Model file for the job. Use its own axes, mm. A direction names the side the tool comes from. Coordinates: 2 decimals unless noted, no trailing zeros. Write each loop counter-clockwise with the first axis right and the second up, starting at its lowest first coordinate (ties: lowest second). Pieces come first, ordered by that corner, then holes. Notation, with made-up numbers: (19.25, 77) - (78.25, 77) arc R27 ccw to (78.25, 109) - close; hole circle Ø7 at (-31.5, 2). An arc over 180 degrees is marked (long way). Put each result on its own line as item: value. Start each with the question number.
1. Saw through at B-B, the plane x = -24. Write the cut outline in (y, z).
2. Which spindle directions (+Z, -Z, +X, -X, +Y, -Y) get a long thin tool onto all of the face, cutting with end or side? Do faces 1 (the face through (2, -7, -5.2)), 2 (the face through (0, 124.252, 0)). Say none if no direction does.
3. Saw through at A-A, the plane z = -3. Write the cut outline in (x, y), plus the area to 3 significant figures.
4. Drill centre lines: L1, parallel to Z at x = 49, y = -55; L2, parallel to X at y = -49, z = -1.75; L3, parallel to X at y = 69.5, z = -2.25. Where is each one in solid material? Low to high. Write a range as from..to.
5. Saw through at C-C, the plane y = 107.5. Write the cut outline in (x, z).
6. Pull direction Z, two halves, no side cores. Call faces 3 (the face through (-79.427, 62.996, 0.08)), 4 (the face through (0, 123.744, 0)), 5 (the face through (-2, -7, 5.708)): released by +Z, released by -Z, zero draft, split by the parting line, or undercut.
7. Drop flat-ended pins along their axis: P1, Ø1, axis at x = -26, z = 3.5, coming from the +Y side; P2, Ø5, axis at x = -104.5, z = -3, coming from the -Y side; P3, Ø0.6, axis at y = 124, z = 4.5, coming from the -X side. Give the stop position or say it passes through.
Autodesk Inventor part; units mm, degrees
ref_plane "YZ Plane" through (0, 0, 0) normal (1, 0, 0) x (0, 1, 0)
ref_plane "XZ Plane" through (0, 0, 0) normal (0, 1, 0) x (-1, 0, 0)
ref_plane "XY Plane" through (0, 0, 0) normal (0, 0, 1) x (1, 0, 0)
sketch "Sketch1" plane through (0, 0, 0) normal (0, 0, 1) x (1, 0, 0)
  line L0 (-141.7042, 0) -> (-17.9605, 123.7437)
  line L1 (17.9605, 123.7437) -> (141.7042, 0)
  line L2 (141.7042, 0) -> (0, -141.7042)
  line L3 (0, -141.7042) -> (-141.7042, 0)
  line L4 (-141.7042, 0) -> (141.7042, 0) construction
  line L5 (0, 141.7042) -> (0, -141.7042) construction
  line L6 (17.9605, 123.7437) -> (-17.9605, 123.7437)
  line L7 (-18.1709, 124.2517) -> (18.1709, 124.2517)
  line L8 (18.1709, 124.2517) -> (142.4226, 0)
  line L9 (142.4226, 0) -> (0, -142.4226)
  line L10 (0, -142.4226) -> (-142.4226, 0)
  line L11 (-142.4226, 0) -> (-18.1709, 124.2517)
  point P0 (0, 0)
  dimension "d0" = 200.4
  dimension "d1" = 200.4
  dimension "d7" = 25.4
  dimension "d8" = 25.4
  dimension "d9" = 0.508
extrude "Extrusion1" add sketch "Sketch1" along normal mid plane 10.4
sketch "Sketch4" plane through (-18.1709, 124.2517, 5.2) normal (0, 1, 0) x (1, 0, 0)
  line L0 (20.1709, 0) -> (16.1709, 0)
  line L1 (16.1709, 0) -> (16.1709, 2)
  line L2 (16.1709, 2) -> (20.1709, 2)
  line L3 (20.1709, 2) -> (20.1709, 0)
  line L4 (36.3419, 0) -> (0, 0)
  point P0 (18.1709, 5.2)
  point P1 (18.1709, 0)
  dimension "d16" = 4
  dimension "d17" = 2
extrude "Extrusion3" cut sketch "Sketch4" against normal up to surface (0.508 mm away)
sketch "Sketch2" plane through (0, 0, 5.2) normal (0, 0, 1) x (1, 0, 0)
  line L0 (142.4226, 0) -> (0, -142.4226)
  line L1 (18.1709, 124.2517) -> (142.4226, 0)
  line L2 (-18.1709, 124.2517) -> (18.1709, 124.2517)
  line L3 (-142.4226, 0) -> (-18.1709, 124.2517)
  line L4 (0, -142.4226) -> (-142.4226, 0)
extrude "Extrusion2" add sketch "Sketch2" along normal blind 0.508
mirror "Mirror1" about plane through (0, 0, 0) normal (0, 0, 1) of "Extrusion2"
equation "\"d0\" = ScintillatorWidth + 2 * silveringThickness"
equation "\"d1\" = ScintillatorHeight + 2 * silveringThickness"
equation "\"d7\" = cornerChamfer"
equation "\"d8\" = d7"
equation "\"d9\" = rubberizedCoating"
equation "\"d3\" = ScintillatorThickness + 2 * silveringThickness"
equation "\"d5\" = rubberizedCoating"
equation "\"OpticalFiberClearence\" = 0.15"
equation "\"ScintillatorEdgeClearence\" = 3"
equation "\"ShallowTrackDepth\" = 1.3"
equation "\"DeepTrackDepth\" = 5.571"
equation "\"FiberEdgeOffsett\" = 5"
equation "\"LoopLargeTrackRatio\" = 1.5"
equation "\"FiberSensorClerence\" = 0.5"
equation "\"MountingScrewOffsett\" = 9"
equation "\"FoilThickness\" = 0.2"
equation "\"silveringThickness\" = 0.2"
equation "\"mppcMountDepth\" = 6.35"
equation "\"opticalFiberClearence\" = 0.071"
equation "\"scintillatorEdgeClearence\" = 3"
equation "\"fiberEdgeOffsett\" = 5"
equation "\"shallowTrackDepth\" = 1.142"
equation "\"deepTrackDepth\" = 5.571"
equation "\"opticalFiberDiameter\" = 1"
equation "\"mountingSpacing\" = 18"
equation "\"cornerChamfer\" = 25.4"
equation "\"SmallTrackDiameter\" = 175"
properties part number "rubberizedCoating" material "Rubber"
Final values:
1. outline: (-118.42, -5.71) - (118.42, -5.71) - (118.42, 5.71) - (-118.42, 5.71) - close; hole (-117.7, -5.2) - (117.7, -5.2) - (117.7, 5.2) - (-117.7, 5.2) - close
2. face 1: none
2. face 2: +Z, -Z, +X, -X, +Y
3. outline: (-142.42, 0) - (0, -142.42) - (142.42, 0) - (18.17, 124.25) - (-18.17, 124.25) - close; hole (-141.7, 0) - (0, -141.7) - (141.7, 0) - (17.96, 123.74) - (-17.96, 123.74) - close
3. area: 401 mm²
4. L1: z = -5.71..-5.2, 5.2..5.71
4. L2: x = -93.42..-92.7, 92.7..93.42
4. L3: x = -72.92..-72.2, 72.2..72.92
5. outline: (-34.92, -5.71) - (34.92, -5.71) - (34.92, 5.71) - (-34.92, 5.71) - close; hole (-34.2, -5.2) - (34.2, -5.2) - (34.2, 5.2) - (-34.2, 5.2) - close
6. face 3: zero draft
6. face 4: undercut
6. face 5: released by +Z
7. P1: stops at y = 116.92
7. P2: stops at y = -40.42
7. P3: stops at x = -18.72
